Check sheet for the modelled part. Datum: model origin and axes. Units: mm. A direction names the side the tool comes from. Coordinates: 2 decimals unless noted, no trailing zeros. Write each loop counter-clockwise with the first axis right and the second up, starting at its lowest first coordinate (ties: lowest second). Pieces come first, ordered by that corner, then holes. Notation, with made-up numbers: (72.5, -4) - (127.5, -4) arc R15 cw to (127.5, 12) - close; hole circle Ø9 at (3.5, -28.75). An arc over 180 degrees is marked (long way). Write each question's results on one line, items separated by ' | '.
from build123d import *

# Parameters (mm, degrees)
F2_SIZE  = 0.5
F3_R     = 1.5
F5_DEPTH = 3


with BuildPart() as f1:
    # F0 (on Front) → F1 (revolve)
    with BuildSketch(Plane.XZ):
        Polygon((-3, 0), (0, 0), (0, 51), (-5, 51), (-5, 45), (-3, 45), align=None)
    revolve(axis=Axis((0, 0, 29.048277), (0, 0, 1)))

    # F2
    f2_edges = [f1.edges().sort_by_distance(p)[0] for p in [
        (3, 0, 0),
    ]]
    chamfer(f2_edges, length=F2_SIZE)

    # F3
    f3_edges = [f1.edges().sort_by_distance(p)[0] for p in [
        (5, 0, 51),
    ]]
    fillet(f3_edges, radius=F3_R)

    # F4 (on face) → F5 (cut)
    with BuildSketch(Plane.XY.offset(51)):
        Polygon((-2, 1.154701), (-2, -1.154701), (0, -2.309401), (2, -1.154701), (2, 1.154701), (0, 2.309401), align=None)
    extrude(amount=-F5_DEPTH, mode=Mode.SUBTRACT)


solid = f1.part
1. Sectioned sample at A-A (y = 0). Record the cut outline in (x, z), then the cut area to 3 significant figures.
Values follow:
outline: (-5, 45) - (-3, 45) - (-3, 0.5) - (-2.5, 0) - (2.5, 0) - (3, 0.5) - (3, 45) - (5, 45) - (5, 49.5) arc R1.5 ccw to (3.5, 51) - (2, 51) - (2, 48) - (-2, 48) - (-2, 51) - (-3.5, 51) arc R1.5 ccw to (-5, 49.5) - close | area: 317 mm^2
2. Material ranges on L1, parallel to Z at x = 0.75, y = 3.5; L2, parallel to Y at x = 4, z = 48; L3, parallel to X at y = 1.75, z = 48.5, recorded low to high. Write a range as [from, to].
Values follow:
L1: z = [45, 51] | L2: y = [-3, 3] | L3: x = [-4.68, -0.97], [0.97, 4.68]
3. Draft check along Y on faces 4 (the flat face through (0, 0, 48)), 5 (the flat face through (2, 2, 51)), 6 (the cylindrical face through (3, 0, 22)). Enter one of: pulls with the +Y half, pulls with the -Y half, needs draft (parallel to the pull), parting line crosses it, or undercut.
Values follow:
face 4: undercut | face 5: needs draft | face 6: parting line crosses it
4. Sectioned sample at B-B (z = 13.5). Record the cut outline in (x, y).
Values follow:
outline: circle Ø6 at (0, 0)
5. Go/stop test with flat-tipped pins: pin 1 (2 mm diameter, centred on x = 3.5, z = 7.5, fed in from -Y); pin 2 (2 mm diameter, centred on x = -1.5, z = 14, fed in from +Y); pin 3 (3 mm diameter, centred on y = -2.5, z = 29, fed in from -X). Record where each tip stops, or that it passes through.
Values follow:
pin 1: stops at y = -1.66 | pin 2: stops at y = 2.96 | pin 3: stops at x = -2.83
6. Access from +Z, -Z, +X, -X, +Y, -Y to the whole of each face (thin tool, end or side, straight path). Record for faces 1 (the flat face through (-3.3, -0.1, 45)), 2 (the cylindrical face through (1.08, 4.88, 47.22)), 3 (the flat face through (2, 0, 50)).
Values follow:
face 1: -Z | face 2: +Z, -Z | face 3: +Z
